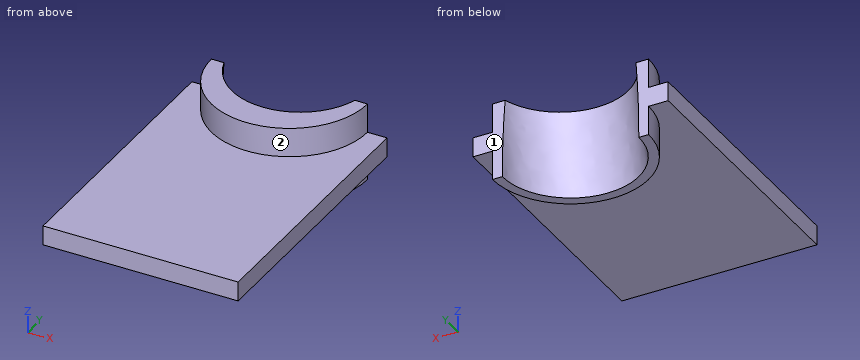
Autodesk Inventor part; units mm, degrees
ref_plane "YZ Plane" through (0, 0, 0) normal (1, 0, 0) x (0, 1, 0)
ref_plane "XZ Plane" through (0, 0, 0) normal (0, 1, 0) x (-1, 0, 0)
ref_plane "XY Plane" through (0, 0, 0) normal (0, 0, 1) x (1, 0, 0)
sketch "草圖1" plane through (0, 0, 0) normal (0, 0, 1) x (1, 0, 0)
  arc A0 (-17.5, 0) -> (17.5, 0) centre (0, 0) ccw
  arc A1 (-20, 0) -> (20, 0) centre (0, 0) ccw
  line L0 (-20, 0) -> (-17.5, 0)
  line L1 (20, 0) -> (17.5, 0)
  line L2 (-35, 0) -> (35, 0)
  line L3 (-25, 0) -> (25, 0)
  line L4 (25, -70) -> (-25, -70)
  line L5 (-25, -70) -> (-25, 0)
  line L6 (-25, 0) -> (25, 0)
  line L7 (25, 0) -> (25, -70)
  line L8 (25, -70) -> (-25, 0) construction
  line L9 (-25, -70) -> (25, 0) construction
  line L10 (0, -84) -> (0, 14)
  point P0 (17.5, 0)
  point P1 (20, 0)
  point P2 (20, 0)
  point P3 (0, -35)
  dimension "d0" = 17.5
  dimension "d16" = 50
  dimension "d17" = 70
  dimension "d22" = 20
extrude "擠出1" add sketch "草圖1" along normal mid plane 20 contours L2 L10 A0 | A0 L10 A1 L0 | L10 L2 A0 | A0 L1 A1 L10
extrude "擠出2" add sketch "草圖1" along normal mid plane 5
sketch "草圖2" plane through (0, 0, 0) normal (1, 0, 0) x (0, 1, 0)
  line L0 (-10, -10) -> (-5, 10)
  line L1 (0, -2.5) -> (0, -10)
  line L2 (0, 10) -> (0, 2.5)
  line L3 (-20, -10) -> (0, -10)
  line L4 (0, 10) -> (-20, 10)
  point P0 (0, 0)
  dimension "d18" = 10
  dimension "d19" = 5
sketch "草圖3" plane through (0, 0, -10) normal (0, 0, -1) x (-1, 0, 0)
  arc A0 (-17.5, 0) -> (17.5, 0) centre (0, 0) ccw
  line L0 (25, 0) -> (-25, 0)
sweep "掃掠1" cut profiles "草圖3" path "草圖2" path curves L0
Check sheet for the modelled part. Datum: model origin and axes. Units: mm. Face numbers are marked on the shaded views. A direction names the side the tool comes from. Round coordinates to 2 decimals unless told otherwise and drop trailing zeros. Order: outer loops, then holes, each group sorted by start corner. A loop starts at its lowest first (then second) coordinate and runs counter-clockwise, first axis right, second up.
1) Scan lines: line 1 (Z direction, x = -14.5, y = -18.5); line 2 (X direction, y = -6, z = -0.5); line 3 (X direction, y = -5.5, z = -1). Record each from-to range of solid material in increasing order.
2) Tool access check on the marked faces 1 and 2. Record the directions out of +Z, -Z, +X, -X, +Y, -Y that give a thin tool (end or side, any length) a straight path to the whole face; none if there is none.
3) Go/stop test with flat-tipped pins: pin 1 Ø1 at (x, y) = (-4.5, -36.5) entering from -Z; pin 2 Ø3 at (x, z) = (-4, 6.5) entering from -Y; pin 3 Ø2 at (y, z) = (-57.5, 4) entering from -X; pin 4 Ø1 at (x, z) = (2, -7) entering from -Y. Record where each tip stops, or that it passes through.
4) Section check B-B (y = -35). Record the boundary of the cut face in (x, z), and give its area (3 significant figures).
5) Section check A-A (x = 18.5). Record the boundary of the cut face in (y, z), and give its area (3 significant figures).
Result:
1. line 1: z = -2.5 to 2.5
1. line 2: x = -25 to -15.37, 15.37 to 25
1. line 3: x = -25 to -15.69, 15.69 to 25
2. face 1: +Z, -Z, +X, -X, +Y
2. face 2: +Z, -Y
3. pin 1: stops at z = -2.5
3. pin 2: stops at y = -19.84
3. pin 3: passes through
3. pin 4: stops at y = -19.94
4. outline: (-25, -2.5) - (25, -2.5) - (25, 2.5) - (-25, 2.5) - close
4. area: 250 mm2
5. outline: (-70, -2.5) - (-7.6, -2.5) - (-7.6, -10) - (0, -10) - (0, 10) - (-7.6, 10) - (-7.6, 2.5) - (-70, 2.5) - close
5. area: 464 mm2
